Build history of the part. All positions in model axes, mm. A direction names the side the tool comes from. Give positions to 0.01 mm unless a question says otherwise; leave off trailing zeros. Loops run counter-clockwise (first coordinate to the right, second up) from the corner with the lowest first, then second, coordinate; pieces in that order, holes last.
1) Band-saw the part on C-C on z = -1.5. List the corners of the cut face in (x, y), then the cut area to 3 significant figures.
2) Two-plate mould, pull along Y, no slides. Class faces 3 (the flat face through (-5.08, -22, 0)), 4 (the cylindrical face through (-8.73, -6.69, 0.04)), 5 (the flat face through (8, -8, 3.175)), 6 (the cylindrical face through (57.598, -0.485, 0.044)): +Y half, -Y half, draft (parallel to the pull), parting line (faces both ways), or undercut.
3) Band-saw the part on A-A on y = 0. List the corners of the cut face in (x, z) (3 decimals).
4) 3-axis set-ups, long thin cutter, end or side, ignore diameter. For faces 1 (the flat face through (8, -8, -3.175)), 2 (the cylindrical face through (9.03, 8.93, 0.04)): which of +Z, -Z, +X, -X, +Y, -Y reach the whole face in a straight line?
5) Flat gauge pins, fed straight in: P1, Ø1.5, axis at y = 29, z = -0.5, coming from the +X side; P2, Ø3, axis at x = 21.5, z = 0, coming from the -Y side; P3, Ø3, axis at y = -12, z = -1.5, coming from the -X side; P4, Ø17.5, axis at x = 0, y = 44.88, coming from the -Z side. Where does each tip first touch, or does it go through?
6) Wall check: line 1 (Y direction, x = 0, z = -1.9); line 2 (X direction, y = 6, z = 0.25); line 3 (Y direction, x = -6, z = 2.25). Give the ranges that are in metal, low to high.
7) Band-saw the part on D-D on y = 28. List the corners of the cut face in (x, z) (3 decimals).
8) Band-saw the part on B-B on x = 0. List the corners of the cut face in (y, z) (3 decimals), then the cut area to 3 significant figures.
```python
from build123d import *

# Parameters (mm, degrees)
F2_DEPTH = 3.175
F1_R     = 10.9982
F3_DEPTH = 3.175


with BuildPart() as f2:
    # F0 (on Top) → F2 (new body, symmetric)
    with BuildSketch(Plane.XY):
        with BuildLine():
            Line((-5.08, 11.6397422652), (-5.08, 9.7567207606))
            Line((-5.08, 9.7567207606), (5.08, 9.7567207606))
            Line((5.08, 9.7567207606), (5.08, 11.6397422652))
            ThreePointArc((5.08, 11.6397422652), (0, 12.7), (-5.08, 11.6397422652))
        make_face()
        with BuildLine():
            Line((5.08, 9.7567207606), (-5.08, 9.7567207606))
            Line((-5.08, 9.7567207606), (-5.08, 11.6397422652))
            ThreePointArc((-5.08, 11.6397422652), (-8.9802561211, 8.9802561211), (-11.6397422652, 5.08))
            Line((-11.6397422652, 5.08), (-9.7536, 5.08))
            Line((-9.7536, 5.08), (-9.7536, -5.08))
            Line((-9.7536, -5.08), (-11.6397422652, -5.08))
            ThreePointArc((-11.6397422652, -5.08), (-8.9802561211, -8.9802561211), (-5.08, -11.6397422652))
            Line((-5.08, -11.6397422652), (-5.08, -9.7536))
            Line((-5.08, -9.7536), (5.08, -9.7536))
            Line((5.08, -9.7536), (5.08, -11.6397422652))
            ThreePointArc((5.08, -11.6397422652), (8.9802561211, -8.9802561211), (11.6397422652, -5.08))
            Line((11.6397422652, -5.08), (9.7536, -5.08))
            Line((9.7536, -5.08), (9.7536, 5.08))
            Line((9.7536, 5.08), (11.6397422652, 5.08))
            ThreePointArc((11.6397422652, 5.08), (8.9802561211, 8.9802561211), (5.08, 11.6397422652))
            Line((5.08, 11.6397422652), (5.08, 9.7567207606))
        make_face()
        with BuildLine():
            Line((-5.08, 33.2674577348), (-5.08, 11.6397422652))
            ThreePointArc((-5.08, 11.6397422652), (0, 12.7), (5.08, 11.6397422652))
            Line((5.08, 11.6397422652), (5.08, 33.2674577348))
            ThreePointArc((5.08, 33.2674577348), (0, 32.2072), (-5.08, 33.2674577348))
        make_face()
        with BuildLine():
            ThreePointArc((12.7, 44.9072), (-6.9560764803, 55.532782337), (-5.08, 33.2674577348))
            Line((-5.08, 33.2674577348), (-5.08, 35.1567207606))
            Line((-5.08, 35.1567207606), (5.08, 35.1567207606))
            Line((5.08, 35.1567207606), (5.08, 33.2674577348))
            ThreePointArc((5.08, 33.2674577348), (10.625582337, 37.9511235197), (12.7, 44.9072))
        make_face()
        with BuildLine():
            Line((-5.08, 35.1567207606), (-5.08, 33.2674577348))
            ThreePointArc((-5.08, 33.2674577348), (0, 32.2072), (5.08, 33.2674577348))
            Line((5.08, 33.2674577348), (5.08, 35.1567207606))
            Line((5.08, 35.1567207606), (-5.08, 35.1567207606))
        make_face()
        with BuildLine():
            ThreePointArc((-11.6397422652, -5.08), (-12.7, 0), (-11.6397422652, 5.08))
            Line((-11.6397422652, 5.08), (-33.2674577348, 5.08))
            ThreePointArc((-33.2674577348, 5.08), (-32.4750898258, 2.5947324749), (-32.2072, 0))
            ThreePointArc((-32.2072, 0), (-32.4750898258, -2.5947324749), (-33.2674577348, -5.08))
            Line((-33.2674577348, -5.08), (-11.6397422652, -5.08))
        make_face()
        with BuildLine():
            Line((-9.7536, 5.08), (-11.6397422652, 5.08))
            ThreePointArc((-11.6397422652, 5.08), (-12.7, 0), (-11.6397422652, -5.08))
            Line((-11.6397422652, -5.08), (-9.7536, -5.08))
            Line((-9.7536, -5.08), (-9.7536, 5.08))
        make_face()
        with BuildLine():
            ThreePointArc((12.7, 0), (12.4321101742, 2.5947324749), (11.6397422652, 5.08))
            Line((11.6397422652, 5.08), (9.7536, 5.08))
            Line((9.7536, 5.08), (9.7536, -5.08))
            Line((9.7536, -5.08), (11.6397422652, -5.08))
            ThreePointArc((11.6397422652, -5.08), (12.4321101742, -2.5947324749), (12.7, 0))
        make_face()
        with BuildLine():
            Line((33.2674577348, 5.08), (11.6397422652, 5.08))
            ThreePointArc((11.6397422652, 5.08), (12.4321101742, 2.5947324749), (12.7, 0))
            ThreePointArc((12.7, 0), (12.4321101742, -2.5947324749), (11.6397422652, -5.08))
            Line((11.6397422652, -5.08), (33.2674577348, -5.08))
            ThreePointArc((33.2674577348, -5.08), (32.2072, 0), (33.2674577348, 5.08))
        make_face()
        with BuildLine():
            ThreePointArc((-32.2072, 0), (-32.4750898258, 2.5947324749), (-33.2674577348, 5.08))
            Line((-33.2674577348, 5.08), (-35.1536, 5.08))
            Line((-35.1536, 5.08), (-35.1536, -5.08))
            Line((-35.1536, -5.08), (-33.2674577348, -5.08))
            ThreePointArc((-33.2674577348, -5.08), (-32.4750898258, -2.5947324749), (-32.2072, 0))
        make_face()
        with BuildLine():
            Line((-35.1536, 5.08), (-33.2674577348, 5.08))
            ThreePointArc((-33.2674577348, 5.08), (-57.6072, 0), (-33.2674577348, -5.08))
            Line((-33.2674577348, -5.08), (-35.1536, -5.08))
            Line((-35.1536, -5.08), (-35.1536, 5.08))
        make_face()
        with BuildLine():
            ThreePointArc((57.6072, 0), (47.5019324749, 12.4321101742), (33.2674577348, 5.08))
            Line((33.2674577348, 5.08), (35.1536, 5.08))
            Line((35.1536, 5.08), (35.1536, -5.08))
            Line((35.1536, -5.08), (33.2674577348, -5.08))
            ThreePointArc((33.2674577348, -5.08), (47.5019324749, -12.4321101742), (57.6072, 0))
        make_face()
        with BuildLine():
            Line((35.1536, 5.08), (33.2674577348, 5.08))
            ThreePointArc((33.2674577348, 5.08), (32.2072, 0), (33.2674577348, -5.08))
            Line((33.2674577348, -5.08), (35.1536, -5.08))
            Line((35.1536, -5.08), (35.1536, 5.08))
        make_face()
        with BuildLine():
            ThreePointArc((5.08, -11.6397422652), (0, -12.7), (-5.08, -11.6397422652))
            Line((-5.08, -11.6397422652), (-5.08, -33.2674577348))
            ThreePointArc((-5.08, -33.2674577348), (0, -32.2072), (5.08, -33.2674577348))
            Line((5.08, -33.2674577348), (5.08, -11.6397422652))
        make_face()
        with BuildLine():
            Line((-5.08, -9.7536), (-5.08, -11.6397422652))
            ThreePointArc((-5.08, -11.6397422652), (0, -12.7), (5.08, -11.6397422652))
            Line((5.08, -11.6397422652), (5.08, -9.7536))
            Line((5.08, -9.7536), (-5.08, -9.7536))
        make_face()
        with BuildLine():
            ThreePointArc((5.08, -33.2674577348), (0, -32.2072), (-5.08, -33.2674577348))
            Line((-5.08, -33.2674577348), (-5.08, -35.1536))
            Line((-5.08, -35.1536), (5.08, -35.1536))
            Line((5.08, -35.1536), (5.08, -33.2674577348))
        make_face()
        with BuildLine():
            Line((-5.08, -35.1536), (-5.08, -33.2674577348))
            ThreePointArc((-5.08, -33.2674577348), (-6.9560764803, -55.532782337), (12.7, -44.9072))
            ThreePointArc((12.7, -44.9072), (10.625582337, -37.9511235197), (5.08, -33.2674577348))
            Line((5.08, -33.2674577348), (5.08, -35.1536))
            Line((5.08, -35.1536), (-5.08, -35.1536))
        make_face()
    extrude(amount=F2_DEPTH, both=True)

    # F1 (on Top) → F3 (cut, symmetric)
    with BuildSketch(Plane.XY):
        with Locations((0, 44.881273061)):
            Circle(F1_R)
        with Locations((44.9082072701, 0)):
            Circle(F1_R)
        with Locations((-44.9071153058, 0)):
            Circle(F1_R)
        with Locations((0, -44.9086768341)):
            Circle(F1_R)
        Circle(F1_R)
    extrude(amount=F3_DEPTH, both=True, mode=Mode.SUBTRACT)


solid = f2.part
```
Findings below:
1. outline: (-33.27, -5.08) - (-11.64, -5.08) arc R12.7 ccw to (-5.08, -11.64) - (-5.08, -33.27) arc R12.7 ccw (long way) to (5.08, -33.27) - (5.08, -11.64) arc R12.7 ccw to (11.64, -5.08) - (33.27, -5.08) arc R12.7 ccw (long way) to (33.27, 5.08) - (11.64, 5.08) arc R12.7 ccw to (5.08, 11.64) - (5.08, 33.27) arc R12.7 ccw (long way) to (-5.08, 33.27) - (-5.08, 11.64) arc R12.7 ccw to (-11.64, 5.08) - (-33.27, 5.08) arc R12.7 ccw (long way) to start; hole circle Ø22 at (-44.91, 0); hole circle Ø22 at (0, -44.91); hole circle Ø22 at (0, 0); hole circle Ø22 at (0, 44.88); hole circle Ø22 at (44.91, 0)
1. area: 1,450 mm2
2. face 3: undercut
2. face 4: undercut
2. face 5: draft
2. face 6: parting line
3. outline: (-57.607, -3.175) - (-55.905, -3.175) - (-55.905, 3.175) - (-57.607, 3.175) - close; (-33.909, -3.175) - (-10.998, -3.175) - (-10.998, 3.175) - (-33.909, 3.175) - close; (10.998, -3.175) - (33.91, -3.175) - (33.91, 3.175) - (10.998, 3.175) - close; (55.906, -3.175) - (57.607, -3.175) - (57.607, 3.175) - (55.906, 3.175) - close
4. face 1: -Z, +X, -X, +Y, -Y
4. face 2: +Z, -Z
5. P1: stops at x = 5.08
5. P2: stops at y = -5.08
5. P3: stops at x = -52.05
5. P4: passes through
6. line 1: y = -57.61 to -55.91, -33.91 to -11, 11 to 33.88, 55.88 to 57.61
6. line 2: x = -56.1 to -54.12, -35.69 to -33.71, -11.19 to -9.22, 9.22 to 11.19, 33.71 to 35.69, 54.13 to 56.1
6. line 3: y = -56.1 to -54.13, -35.69 to -33.71, -11.19 to -9.22, 9.22 to 11.19, 33.71 to 35.66, 54.1 to 56.1
7. outline: (-5.08, -3.175) - (5.08, -3.175) - (5.08, 3.175) - (-5.08, 3.175) - close
8. outline: (-57.607, -3.175) - (-55.907, -3.175) - (-55.907, 3.175) - (-57.607, 3.175) - close; (-33.91, -3.175) - (-10.998, -3.175) - (-10.998, 3.175) - (-33.91, 3.175) - close; (10.998, -3.175) - (33.883, -3.175) - (33.883, 3.175) - (10.998, 3.175) - close; (55.879, -3.175) - (57.607, -3.175) - (57.607, 3.175) - (55.879, 3.175) - close
8. area: 313 mm2
